Here's how the part is built. I have some questions about the finished solid (model axes, mm). Face numbers are marked on the shaded views. A direction names the side the tool comes from. Coordinates: 2 decimals unless noted, no trailing zeros. Loops run counter-clockwise (first coordinate to the right, second up) from the corner with the lowest first, then second, coordinate; pieces in that order, holes last. Notation, with made-up numbers: (53, 64) -> (72, 64) arc R18 ccw to (72, 91) -> close; hole circle Ø4 at (13, -0.5). An arc over 180 degrees is marked (long way). Use CSV: the item, a comma, the result in double quotes. Start each with the question number.
from build123d import *

# Parameters (mm, degrees)
BOSS_EXTRUDE1_DEPTH     = 100
SKETCH3_R               = 6
BOSS_EXTRUDE2_DEPTH     = 4
BOSS_EXTRUDE3_START     = 4
SKETCH4_R               = 6
BOSS_EXTRUDE3_DEPTH     = 4
CUT_EXTRUDE1_DEPTH      = 130.646635128
CUT_EXTRUDE1_DEPTH_BACK = 130.646635128
SKETCH9_R               = 4.1
CUT_EXTRUDE2_DEPTH      = 134.341666406
CUT_EXTRUDE2_DEPTH_BACK = 134.341666406
SKETCH10_R              = 2.55
SKETCH13_W              = 60
SKETCH13_H              = 31.00370213
CUT_EXTRUDE5_DEPTH      = 24
FILLET1_R               = 3
FILLET2_R               = 5
FILLET3_R               = 4
SKETCH15_R              = 2.15
CUT_EXTRUDE6_DEPTH      = 132.954537626


with BuildPart() as part:
    # Sketch2 → Boss-Extrude1 (new body)
    with BuildSketch(Plane.XY):
        Polygon((0, 0), (0, 23.99629787), (7.5, 38), (7.5, 70), (32.5, 70), (32.5, 38), (40, 23.99629787), (40, 0), (44, 0), (44, 25), (36.5, 39.00370213), (36.5, 74), (3.5, 74), (3.5, 39.00370213), (-4, 25), (-4, 0), align=None)
    extrude(amount=BOSS_EXTRUDE1_DEPTH)

    # Sketch3 → Boss-Extrude2 (add)
    with BuildSketch(Plane.ZY.offset(-32.5)):
        with Locations(Location((84, 46, 0), (0, 0, 90))):
            Circle(SKETCH3_R)
        with Locations(Location((16, 46, 0), (0, 0, 90))):
            Circle(SKETCH3_R)
    extrude(amount=BOSS_EXTRUDE2_DEPTH)

    # Sketch4 → Boss-Extrude3 (add)
    with BuildSketch(Plane(origin=(7.5, 0, 0), x_dir=(0, 0, -1), z_dir=(1, 0, 0)).offset(BOSS_EXTRUDE3_START)):
        with Locations(Location((-16, 46, 0), (0, 0, 90))):
            Circle(SKETCH4_R)
        with Locations(Location((-84, 46, 0), (0, 0, 90))):
            Circle(SKETCH4_R)
    extrude(amount=-BOSS_EXTRUDE3_DEPTH)

    # Sketch9 → Cut-Extrude1 (cut, two sides: drawn at the far end of the back side and taken through both)
    with BuildSketch(Plane(origin=(7.5, 0, 0), x_dir=(0, 0, -1), z_dir=(1, 0, 0)).offset(-CUT_EXTRUDE1_DEPTH_BACK)):
        with Locations((-16, 46)):
            Circle(SKETCH9_R)
        with Locations((-84, 46)):
            Circle(SKETCH9_R)
    extrude(amount=CUT_EXTRUDE1_DEPTH + CUT_EXTRUDE1_DEPTH_BACK, mode=Mode.SUBTRACT)

    # Sketch10 → Cut-Extrude2 (cut, two sides: drawn at the far end of the back side and taken through both)
    with BuildSketch(Plane(origin=(44, 0, 0), x_dir=(0, 0, -1), z_dir=(1, 0, 0)).offset(-CUT_EXTRUDE2_DEPTH_BACK)):
        with Locations(Location((-10, 10, 0), (0, 0, 90))):
            Circle(SKETCH10_R)
        with Locations(Location((-90, 10, 0), (0, 0, 90))):
            Circle(SKETCH10_R)
    extrude(amount=CUT_EXTRUDE2_DEPTH + CUT_EXTRUDE2_DEPTH_BACK, mode=Mode.SUBTRACT)

    # Sketch13 → Cut-Extrude5 (cut)
    with BuildSketch(Plane.ZY.offset(4)):
        with Locations((50, 15.501851065)):
            Rectangle(SKETCH13_W, SKETCH13_H)
    extrude(amount=-CUT_EXTRUDE5_DEPTH, mode=Mode.SUBTRACT)

    # Fillet1
    fillet1_edges = [part.edges().sort_by_distance(p)[0] for p in [
        (1.48419643, 31.00370213, 20),
        (1.48419643, 31.00370213, 80),
    ]]
    fillet(fillet1_edges, radius=FILLET1_R)

    # Fillet2
    fillet2_edges = [part.edges().sort_by_distance(p)[0] for p in [
        (32.5, 70, 50),
        (7.5, 70, 50),
    ]]
    fillet(fillet2_edges, radius=FILLET2_R)

    # Fillet3
    fillet3_edges = [part.edges().sort_by_distance(p)[0] for p in [
        (-4, 25, 10),
        (0, 23.99629787, 10),
        (-4, 25, 90),
        (3.5, 39.00370213, 50),
        (36.5, 39.00370213, 50),
        (44, 25, 50),
        (40, 23.99629787, 50),
        (32.5, 38, 50),
        (7.5, 38, 50),
        (0, 23.99629787, 90),
    ]]
    fillet(fillet3_edges, radius=FILLET3_R)

    # Sketch15 → Cut-Extrude6 (cut, through all)
    with BuildSketch(Plane(origin=(0, 74, 0), x_dir=(1, 0, 0), z_dir=(0, 1, 0))):
        with Locations(Location((20, -20, 0), (0, 0, 270))):
            Circle(SKETCH15_R)
        with Locations(Location((20, -80, 0), (0, 0, 270))):
            Circle(SKETCH15_R)
    extrude(amount=-CUT_EXTRUDE6_DEPTH, mode=Mode.SUBTRACT)


solid = part.part
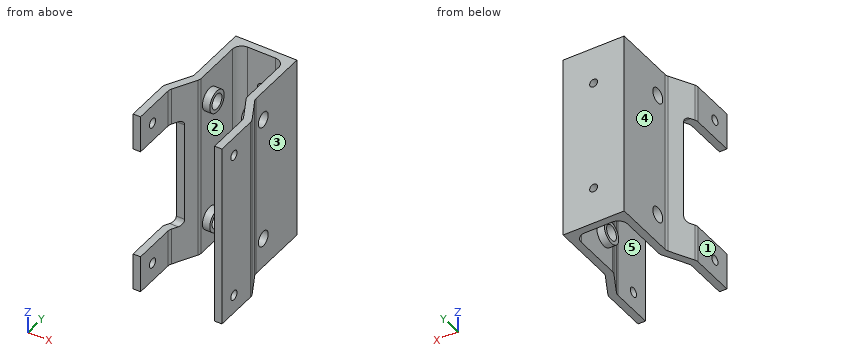
1) I want a section at C-C, the plane y = 20.5. Please give me the cut outline in (x, z).
2) I want a section at D-D, the plane z = 58.5. Please give me the cut outline in (x, y).
3) Which directions (+Z, -Z, +X, -X, +Y, -Y) give clear straight access to the entire face, cutting with the end or side of a thin tool? Please do the marked faces 3, 4 and 5.
4) I want a section at B-B, the plane x = 20. Please give me the cut outline in (y, z), plus the area to 3 significant figures.
5) Please list where these lines run through material, in increasing order: L1, parallel to Z at x = 6.5, y = 46; L2, parallel to Z at x = 30, y = 46; L3, parallel to Z at x = 41.05, y = 10. Write a range as [from, to].
6) I want a section at A-A, the plane y = 10. Please give me the cut outline in (x, z).
7) For P1, Ø3.5, axis at y = 49, z = 82.5, coming from the +X side; P2, Ø10.5, axis at y = 46, z = 16, coming from the -X side; P3, Ø1, axis at y = 29, z = 27.5, coming from the -X side, each with a flat end and sliding along its axis, tell me the tip position at first contact or that it passes through.
8) Thinking about a two-plate mould opening in Z: for the marked faces 1 and 2, which applies, pulls with the +Z half, pulls with the -Z half, needs draft (parallel to the pull), parting line crosses it, or undercut?
Return value:
1,outline,"(-4, 0) -> (0, 0) -> (0, 20) -> (-4, 20) -> close; (-4, 80) -> (0, 80) -> (0, 100) -> (-4, 100) -> close; (40, 0) -> (44, 0) -> (44, 100) -> (40, 100) -> close"
2,outline,"(-0.78, 31) -> (3.75, 31) -> (7.03, 37.12) arc R4 ccw to (7.5, 39) -> (7.5, 65) arc R5 cw to (12.5, 70) -> (27.5, 70) arc R5 cw to (32.5, 65) -> (32.5, 39) arc R4 ccw to (32.97, 37.12) -> (39.53, 24.88) arc R4 cw to (40, 22.99) -> (40, 0) -> (44, 0) -> (44, 24) arc R4 ccw to (43.53, 25.88) -> (36.97, 38.12) arc R4 cw to (36.5, 40.01) -> (36.5, 74) -> (3.5, 74) -> (3.5, 40.01) arc R4 cw to (3.03, 38.12) -> close"
3,face 3,"+Z, -Z, +X, +Y"
3,face 4,"+Z, -Z, -X, +Y"
3,face 5,"+Z, -Z, -Y"
4,outline,"(70, 0) -> (74, 0) -> (74, 17.85) -> (70, 17.85) -> close; (70, 22.15) -> (74, 22.15) -> (74, 77.85) -> (70, 77.85) -> close; (70, 82.15) -> (74, 82.15) -> (74, 100) -> (70, 100) -> close"
4,area,"366 mm²"
5,L1,"z = [0, 11.9], [20.1, 79.9], [88.1, 100]"
5,L2,"z = [10, 11.9], [20.1, 22], [78, 79.9], [88.1, 90]"
5,L3,"z = [0, 7.45], [12.55, 87.45], [92.55, 100]"
6,outline,"(-4, 0) -> (0, 0) -> (0, 7.45) -> (-4, 7.45) -> close; (-4, 12.55) -> (0, 12.55) -> (0, 20) -> (-4, 20) -> close; (-4, 80) -> (0, 80) -> (0, 87.45) -> (-4, 87.45) -> close; (-4, 92.55) -> (0, 92.55) -> (0, 100) -> (-4, 100) -> close; (40, 0) -> (44, 0) -> (44, 7.45) -> (40, 7.45) -> close; (40, 12.55) -> (44, 12.55) -> (44, 87.45) -> (40, 87.45) -> close; (40, 92.55) -> (44, 92.55) -> (44, 100) -> (40, 100) -> close"
7,P1,"stops at x = 36.5"
7,P2,"stops at x = 3.5"
7,P3,"stops at x = 37.05"
8,face 1,"needs draft"
8,face 2,"undercut"
